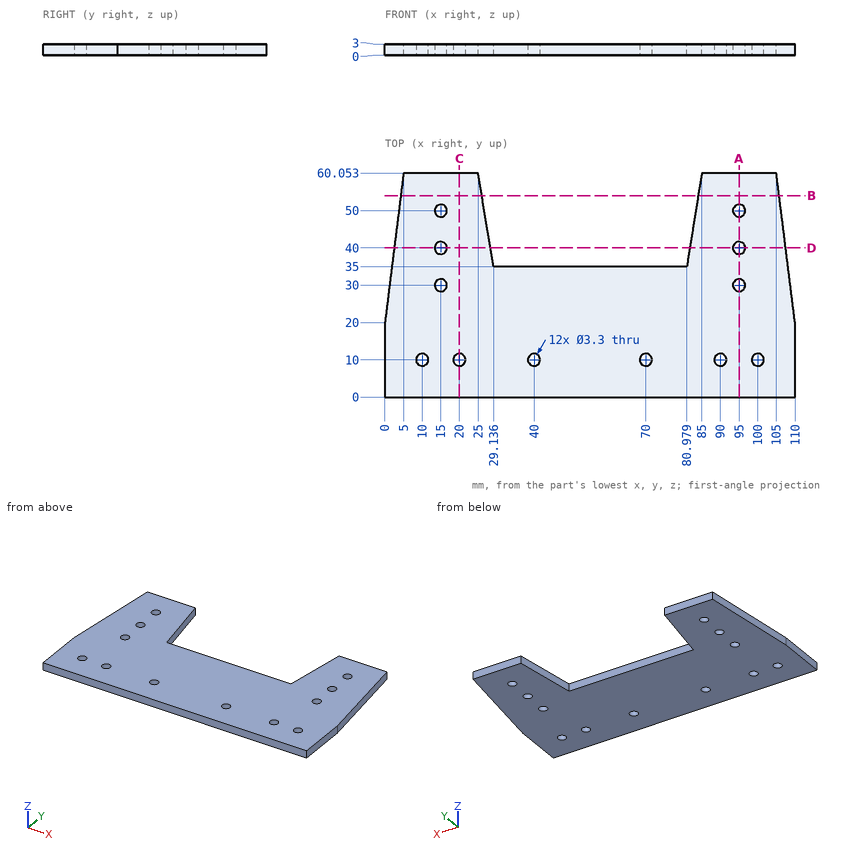
Source: three-view drawing plus pictorial views. Frame: mm from the lowest corner of the part. Round coordinates to 2 decimals unless told otherwise and drop trailing zeros. Write each loop counter-clockwise with the first axis right and the second up, starting at its lowest first coordinate (ties: lowest second). Pieces come first, ordered by that corner, then holes. Notation, with made-up numbers: M 41.25,-37.5 L 64.25,-37.5 A21 ccw 64.25,-31.5 Z; hole C 85.25,-35.5 d11. An arc over 180 degrees is marked long. Use CSV: the item, a comma, the result in double quotes. Start each with the question number.
Q1. Line query: line 1 (Y direction, x = 95, z = 2.4); line 2 (Y direction, x = 10, z = 1.25); line 3 (Y direction, x = 36.5, z = 2.1). Output: solid intervals per line, ascending. Write a range as from..to.
Q2. First-contact query: P1, Ø2.5, axis at x = 15, y = 30, coming from the +Z side; P2, Ø2, axis at x = 12, y = 35, coming from the -Z side. Flat tips, straight axial feed; report the tip coordinate or a pass-through.
Q3. Cut plane D-D on y = 40. Output: boundary loops of the cut face in (x, z), plus the area to 3 significant figures.
Q4. Cut plane A-A on x = 95. Output: boundary loops of the cut face in (y, z).
Q5. Cut plane C-C on x = 20. Output: boundary loops of the cut face in (y, z), plus the area to 3 significant figures.
Q6. Cut plane B-B on y = 54. Output: boundary loops of the cut face in (x, z) (1 decimal).
Results found:
1,line 1,"0..28.35, 31.65..38.35, 41.65..48.35, 51.65..60.05"
1,line 2,"0..8.35, 11.65..60.05"
1,line 3,"0..35"
2,P1,"through"
2,P2,"z = 0"
3,outline,"M 2.5,0 L 13.35,0 L 13.35,3 L 2.5,3 Z; M 16.65,0 L 28.31,0 L 28.31,3 L 16.65,3 Z; M 81.78,0 L 93.35,0 L 93.35,3 L 81.78,3 Z; M 96.65,0 L 107.5,0 L 107.5,3 L 96.65,3 Z"
3,area,"135 mm^2"
4,outline,"M 0,0 L 28.35,0 L 28.35,3 L 0,3 Z; M 31.65,0 L 38.35,0 L 38.35,3 L 31.65,3 Z; M 41.65,0 L 48.35,0 L 48.35,3 L 41.65,3 Z; M 51.65,0 L 60.05,0 L 60.05,3 L 51.65,3 Z"
5,outline,"M 0,0 L 8.35,0 L 8.35,3 L 0,3 Z; M 11.65,0 L 60.05,0 L 60.05,3 L 11.65,3 Z"
5,area,"170 mm^2"
6,outline,"M 4.2,0 L 26,0 L 26,3 L 4.2,3 Z; M 84,0 L 105.8,0 L 105.8,3 L 84,3 Z"
